Can you work these out from the model? Positions are in its coordinate system, mm. Face numbers are marked on the shaded views. A direction names the side the tool comes from. Give positions to 0.01 mm unless a question says otherwise; leave off trailing zeros. Loops run counter-clockwise (first coordinate to the right, second up) from the corner with the lowest first, then second, coordinate; pieces in that order, holes last.
from build123d import *

# Parameters (mm, degrees)
F1_DEPTH = 12.7
F3_DEPTH = 63.5
F4_W     = 13.838368
F4_H     = 6.35
F5_DEPTH = 50.8


with BuildPart() as f1:
    # F0 (on Top) → F1 (new body)
    with BuildSketch(Plane.XY):
        Polygon((0, -76.2), (0, 0), (-76.2, 0), (-76.2, -76.2), (-69.85, -76.2), (-69.85, -6.35), (-38.1, -6.35), (-6.35, -6.35), (-6.35, -38.1), (-6.35, -76.2), align=None)
    extrude(amount=F1_DEPTH)

    # F2 (on face) → F3 (join)
    with BuildSketch(Plane.YZ.offset(-69.85)):
        Polygon((-76.2, 0), (-6.35, 0), (-6.35, 6.35), align=None)
    extrude(amount=F3_DEPTH)

    # F4 (on face) → F5 (join)
    with BuildSketch(Plane.XY.offset(12.7)):
        with Locations((-38.1, -3.175)):
            Rectangle(F4_W, F4_H)
    extrude(amount=F5_DEPTH)


solid = f1.part
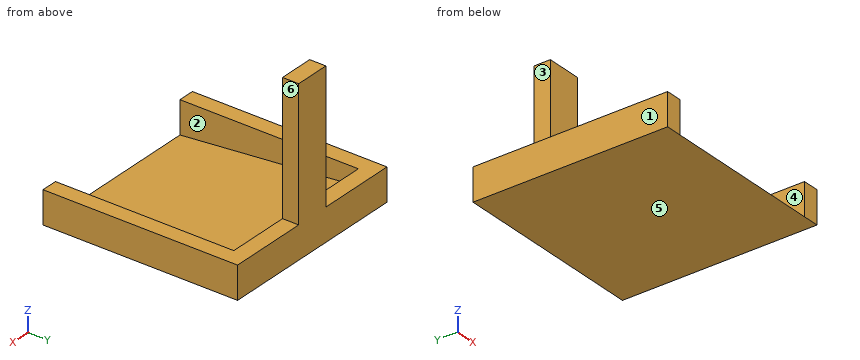
(1) Suppose I cut it at D-D on z = 41.5. List the corners of the cut face in (x, y) for me.
Returned:
outline: (-45.02, -6.35) - (-31.18, -6.35) - (-31.18, 0) - (-45.02, 0) - close
(2) Suppose I cut it at C-C on y = -51.5. List the corners of the cut face in (x, z) for me, plus the area to 3 significant figures.
Returned:
outline: (-76.2, 0) - (0, 0) - (0, 12.7) - (-6.35, 12.7) - (-6.35, 2.25) - (-69.85, 2.25) - (-69.85, 12.7) - (-76.2, 12.7) - close
area: 304 mm2
(3) Will these pins go through, and if not, where does the flat tip stop? P1, Ø3, axis at y = -3.5, z = 47.5, coming from the -X side; P2, Ø12, axis at x = -57, y = -67.5, coming from the +Z side; P3, Ø8, axis at x = -33.5, y = -67, coming from the +Z side.
Returned:
P1: stops at x = -45.02
P2: stops at z = 1.34
P3: stops at z = 1.2
(4) Please list where these lines run through material, in increasing order: probe 1 along X at (y, z) = (-6.5, 11); probe 2 along Z at (x, y) = (-4.5, -30); probe 3 along Y at (x, z) = (-32, 58.5).
Returned:
probe 1: x = -76.2 to -69.85, -6.35 to 0
probe 2: z = 0 to 12.7
probe 3: y = -6.35 to 0
(5) Suppose I cut it at B-B on z = 8.5. List the corners of the cut face in (x, y) for me.
Returned:
outline: (-76.2, -76.2) - (-69.85, -76.2) - (-69.85, -6.35) - (-6.35, -6.35) - (-6.35, -76.2) - (0, -76.2) - (0, 0) - (-76.2, 0) - close
(6) Which directions (+Z, -Z, +X, -X, +Y, -Y) give clear straight access to the entire face, cutting with the end or side of a thin tool? Please do the marked faces 1, 2 and 3.
Returned:
face 1: +Z, -Z, -X, +Y, -Y
face 2: +Z, -Y
face 3: +Z, -X, +Y, -Y
(7) Thinking about a two-plate mould opening in X: for the marked faces 4, 5 and 6, which applies, pulls with the +X half, pulls with the -X half, needs draft (parallel to the pull), parting line crosses it, or undercut?
Returned:
face 4: undercut
face 5: needs draft
face 6: pulls with the +X half
(8) Suppose I cut it at A-A on x = -27. List the corners of the cut face in (y, z) for me.
Returned:
outline: (-76.2, 0) - (0, 0) - (0, 12.7) - (-6.35, 12.7) - (-6.35, 6.35) - close
